The listing builds one solid part. Answer for the finished solid, in the listing's coordinates (mm). A direction names the side the tool comes from. Coordinates: 2 decimals unless noted, no trailing zeros. Order: outer loops, then holes, each group sorted by start corner. A loop starts at its lowest first (then second) coordinate and runs counter-clockwise, first axis right, second up. Notation, with made-up numbers: (-36, -34.75) -> (10, -34.75) arc R21 cw to (10, -8.75) -> close; hole circle Ø6 at (37.25, -14). An arc over 180 degrees is marked (long way). Write item = value, one per line.
from build123d import *

# Parameters (mm, degrees)
SKETCH2_R           = 1.6
BOSS_EXTRUDE1_DEPTH = 2
CHAMFER1_SIZE       = 16
CHAMFER1_SIZE2      = 16.908072044
CUT_EXTRUDE1_DEPTH  = 2
CUT_EXTRUDE2_DEPTH  = 2
FILLET1_R           = 3
FILLET2_R           = 1.5
SKETCH5_R           = 1.6
CUT_EXTRUDE3_DEPTH  = 2


with BuildPart() as part:
    # Sketch2 → Boss-Extrude1 (new body)
    with BuildSketch(Plane.XY):
        Polygon((20.342311206, 18.763435595), (67.83529335, 73.163119739), (108.3419511, 64.404376963), (148.006657298, 9.405462998), (142.666805642, -15.289809939), (75.921402075, -58.302296892), align=None)
        with Locations((25.032859693, 16.533479235)):
            Circle(SKETCH2_R, mode=Mode.SUBTRACT)
        with Locations((66.656313732, 64.210054816)):
            Circle(SKETCH2_R, mode=Mode.SUBTRACT)
        with Locations((134.6128014, 6.607635241)):
            Circle(SKETCH2_R, mode=Mode.SUBTRACT)
        Polygon((140.259166073, -10.893068121), (140.856941108, -8.128531088), (95.641730286, 62.034989033), (78.595202191, 65.720954825), (31.596135929, 11.887014645), (63.750974908, -38.009837557), (74.675087949, -53.157166528), align=None, mode=Mode.SUBTRACT)
    extrude(amount=BOSS_EXTRUDE1_DEPTH)

    # Chamfer1
    chamfer1_edges = [part.edges().sort_by_distance(p)[0] for p in [
        (74.675087949, -53.157166528, 1),
    ]]
    chamfer1_side = [part.faces().sort_by_distance(p)[0] for p in [
        (107.467127011, -32.025117325, 1),
    ]]
    chamfer(chamfer1_edges, length=CHAMFER1_SIZE, length2=CHAMFER1_SIZE2, reference=chamfer1_side[0])

    # Sketch3 → Cut-Extrude1 (cut)
    with BuildSketch(Plane.XY.offset(2)):
        Polygon((67.984533977, -47.297069134), (86.714380981, -51.347018482), (75.921402075, -58.302296892), align=None)
    extrude(amount=-CUT_EXTRUDE1_DEPTH, mode=Mode.SUBTRACT)

    # Sketch4 → Cut-Extrude2 (cut)
    with BuildSketch(Plane.XY.offset(2)):
        Polygon((25.857368283, 20.518945125), (30.060999178, 14.690208293), (69.985569717, 60.420838986), (62.168846417, 62.111046782), align=None)
        Polygon((102.03518682, 62.698754981), (106.582335629, 61.715526322), (144.792131882, 8.733984336), (142.787091436, -0.538749114), align=None)
    extrude(amount=-CUT_EXTRUDE2_DEPTH, mode=Mode.SUBTRACT)

    # Fillet1
    fillet1_edges = [part.edges().sort_by_distance(p)[0] for p in [
        (78.595202191, 65.720954825, 1),
        (95.641730286, 62.034989033, 1),
        (88.124336223, -44.490118537, 1),
        (25.857368283, 20.518945125, 1),
        (62.168846417, 62.111046782, 1),
        (69.985569717, 60.420838986, 1),
        (30.060999178, 14.690208293, 1),
        (142.787091436, -0.538749114, 1),
        (106.582335629, 61.715526322, 1),
        (144.792131882, 8.733984336, 1),
    ]]
    fillet(fillet1_edges, radius=FILLET1_R)

    # Fillet2
    fillet2_edges = [part.edges().sort_by_distance(p)[0] for p in [
        (102.03518682, 62.698754981, 1),
    ]]
    fillet(fillet2_edges, radius=FILLET2_R)

    # Sketch5 → Cut-Extrude3 (cut)
    with BuildSketch(Plane.XY.offset(2)):
        with Locations((75.149933369, -45.265554274)):
            Circle(SKETCH5_R)
    extrude(amount=-CUT_EXTRUDE3_DEPTH, mode=Mode.SUBTRACT)


solid = part.part
Q1. Section C-C, the plane y = 24 is taken. Give the vertices of the cut face in (x, z), plus the area to 3 significant figures.
The answers:
outline = (24.91, 0) -> (28.9, 0) -> (28.9, 2) -> (24.91, 2) -> close; (38.19, 0) -> (42.17, 0) -> (42.17, 2) -> (38.19, 2) -> close; (120.15, 0) -> (126.97, 0) -> (126.97, 2) -> (120.15, 2) -> close; (133.78, 0) -> (137.48, 0) -> (137.48, 2) -> (133.78, 2) -> close
area = 37.0 mm2
Q2. Find the intervals of material crossed by line 1 along X through (y, z) = (54.5, 1.55); line 2 along X through (y, z) = (35.5, 0.65); line 3 along Y through (x, z) = (108, 1.7), in increasing order.
The answers:
line_1 = 51.54 to 55.52, 64.82 to 68.8, 100.5 to 107.32, 111.79 to 115.48
line_2 = 34.95 to 38.94, 48.23 to 52.21, 112.74 to 119.56, 125.49 to 129.19
line_3 = -37.63 to -31.68, 42.86 to 53.44, 59.75 to 64.48
Q3. Section A-A, the plane y = -25 is taken. Give the vertices of the cut face in (x, z).
The answers:
outline = (51.9, 0) -> (55.37, 0) -> (55.37, 2) -> (51.9, 2) -> close; (118.37, 0) -> (127.6, 0) -> (127.6, 2) -> (118.37, 2) -> close
Q4. Section B-B, the plane x = 125 is taken. Give the vertices of the cut face in (y, z), plus the area to 3 significant figures.
The answers:
outline = (-26.67, 0) -> (-20.73, 0) -> (-20.73, 2) -> (-26.67, 2) -> close; (16.48, 0) -> (27.06, 0) -> (27.06, 2) -> (16.48, 2) -> close; (36.18, 0) -> (41.31, 0) -> (41.31, 2) -> (36.18, 2) -> close
area = 43.3 mm2
Q5. A tool of negligible diameter and unlimited length cuts with its end or side. For faces 1 (the face through (118, 30, 2)), 2 (the face through (47.448, -12.712, 0.986)), from which of +Z, -Z, +X, -X, +Y, -Y can it reach the whole face along a straight path? Write none if from no direction.
The answers:
face_1 = +Z, +X, -X, +Y, -Y
face_2 = +Z, -Z
Q6. The mould has two halves that part along Y. Classify faces 3 (the face through (43.756, 45.582, 0.986)), 4 (the face through (73.55, -45.2, 1.01)), 5 (the face through (44.497, -14.729, 0.986)): released by +Y, released by -Y, zero draft, split by the parting line, or undercut.
The answers:
face_3 = released by +Y
face_4 = undercut
face_5 = released by -Y
Q7. Section D-D, the plane x = 84 is taken. Give the vertices of the cut face in (y, z), plus the area to 3 significant figures.
The answers:
outline = (-50.76, 0) -> (-43.6, 0) -> (-43.6, 2) -> (-50.76, 2) -> close; (64.55, 0) -> (69.67, 0) -> (69.67, 2) -> (64.55, 2) -> close
area = 24.6 mm2
